Geometry check sheet. Reference: the model listing, model coordinates, mm. A direction names the side the tool comes from. Round coordinates to 2 decimals unless told otherwise and drop trailing zeros. Order: outer loops, then holes, each group sorted by start corner. A loop starts at its lowest first (then second) coordinate and runs counter-clockwise, first axis right, second up. Notation, with made-up numbers: (24, -6) - (58, -6) arc R17 cw to (58, 9) - close; hole circle Ø8 at (12, -30). An arc over 180 degrees is marked (long way). Use a Markdown table: item, result. Add a question column.
(1) Access from +Z, -Z, +X, -X, +Y, -Y to the whole of each face (thin tool, end or side, straight path). Record for faces 4 (the face through (-75, 265, -13)), 5 (the face through (81, 240, 0)), 6 (the face through (0, 227.9, -36.2)).
(2) Gauge pin test, flat ends, axial feed: P1, Ø8, axis at x = -54.5, y = 228, coming from the -Z side; P2, Ø5, axis at x = -38, z = -19, coming from the -Y side; P3, Ø2, axis at x = 63.5, z = -19.5, coming from the -Y side. Record the tip position at first contact, or that the pin passes through.
(3) Section check A-A on x = 45. Record the boundary of the cut face in (y, z), then the cut area to 3 significant figures.
(4) Thickness scan on line 1 along Y through (x, z) = (58.5, 0); line 2 along Y through (x, z) = (53, -24); line 3 along X through (y, z) = (245, 7.5). Record the ranges inside material, lowest first. Write a range as [from, to].
(5) Mould release check, pull along X, two halves, no side actions. Record for faces 1 (the face through (86, 240, -1)), 2 (the face through (38.602, 272.343, 7.154)), 3 (the face through (42.398, 277.224, 8.238)): released by +X, released by -X, zero draft, split by the parting line, or undercut.
```python
from build123d import *


with BuildPart() as part:
    # Sketch1 → Revolve1 (revolve)
    with BuildSketch(Plane.XY, mode=Mode.PRIVATE) as revolve1_sk:
        with BuildLine():
            Line((0, 278.127906977), (0, 280.627906977))
            ThreePointArc((0, 280.627906977), (-37.845738323, 278.064241255), (-75, 270.420084635))
            Line((-75, 270.420084635), (-75, 267.824817071))
            ThreePointArc((-75, 267.824817071), (-40.327501461, 275.188708462), (-5, 278.082959994))
            Line((-5, 278.082959994), (-5, 273.127906977))
            Line((-5, 273.127906977), (81, 273.127906977))
            Line((81, 273.127906977), (81, 245.127906977))
            Line((81, 245.127906977), (81, 240.127906977))
            Line((81, 240.127906977), (86, 240.127906977))
            Line((86, 240.127906977), (86, 278.127906977))
            Line((86, 278.127906977), (0, 278.127906977))
        make_face()
    revolve(revolve1_sk.sketch.rotate(Axis((-150, 240.127906977, 0), (-1, 0, 0)), 90), axis=Axis((-150, 240.127906977, 0), (-1, 0, 0)))


solid = part.part
```
Check sheet entries:
| question | item | result |
|---|---|---|
| 1 | face 4 | +Z, -Z, -X, +Y, -Y |
| 1 | face 5 | none |
| 1 | face 6 | +X |
| 2 | P1 | stops at z = -34.48 |
| 2 | P2 | stops at y = 205.93 |
| 2 | P3 | stops at y = 206.94 |
| 3 | outline | circle Ø76 at (240.13, 0); hole circle Ø66 at (240.13, 0) |
| 3 | area | 1,120 mm2 |
| 4 | line 1 | y = [202.13, 207.13], [273.13, 278.13] |
| 4 | line 2 | y = [210.67, 217.48], [262.78, 269.59] |
| 4 | line 3 | x = [81, 86] |
| 5 | face 1 | released by +X |
| 5 | face 2 | undercut |
| 5 | face 3 | zero draft |
